The listing builds one solid part. Answer for the finished solid, in the listing's coordinates (mm). Coordinates: 2 decimals unless noted, no trailing zeros. Loops run counter-clockwise (first coordinate to the right, second up) from the corner with the lowest first, then second, coordinate; pieces in that order, holes last. Notation, with made-up numbers: (-21.5, -22.75) - (27.5, -22.75) arc R23 cw to (27.5, 5.25) - close; hole circle Ø7 at (59, -7). An arc over 180 degrees is marked (long way). Return JSON: item names as keys, results as strings. Group by question number.
1. Section B-B (y = 234.5) is taken. Write down the section's boundary in (x, z), and give its area (3 significant figures).
2. Find the intervals of material crossed by line 1 along Y through (x, z) = (152.5, 5); line 2 along X through (y, z) = (35, 3.75); line 3 along Y through (x, z) = (40, 4), in increasing order.
3. Section A-A (z = 6.5) is taken. State how many separate pieces and enclosed holes the cut face has, and give its area (3 significant figures).
4. Section C-C (x = 331) is taken. Write down the section's boundary in (y, z).
5. Each of these flat-tipped pins is pushed along its axis until it touches: P1, Ø3, axis at x = 231.5, z = 6.5, coming from the +Y side; P2, Ø2, axis at x = 375.5, z = 11, coming from the +Y side; P3, Ø6, axis at y = 74, z = 5, coming from the +X side. Where does it stop, or does it pass through?
```python
from build123d import *

# Parameters (mm, degrees)
F1_DEPTH = 12.7
F3_DEPTH = 12.701
F5_D     = 5.08


with BuildPart() as f1:
    # F0 (on Top) → F1 (new body)
    with BuildSketch(Plane.XY):
        Polygon((349.925731, -349.925731), (494.869714, 0), (349.925731, 349.925731), (0, -494.869714), align=None)
    extrude(amount=F1_DEPTH)

    # F2 (on face) → F3 (cut, through all)
    with BuildSketch(Plane.XY.offset(12.7)):
        with BuildLine():
            Line((357.632779, 298.132571), (354.903108, 299.75415))
            ThreePointArc((354.903108, 299.75415), (356.79197, 295.070926), (360.807779, 298.132571))
            ThreePointArc((360.807779, 298.132571), (360.746772, 298.751982), (360.566096, 299.347591))
            Line((360.566096, 299.347591), (357.632779, 298.132571))
        make_face()
        with BuildLine():
            ThreePointArc((360.566096, 299.347591), (357.860135, 301.29942), (354.903108, 299.75415))
            Line((354.903108, 299.75415), (357.632779, 298.132571))
            Line((357.632779, 298.132571), (360.566096, 299.347591))
        make_face()
        with BuildLine():
            Line((463.696126, 42.073001), (463.696126, 45.248001))
            ThreePointArc((463.696126, 45.248001), (461.451062, 39.827937), (466.871126, 42.073001))
            ThreePointArc((466.871126, 42.073001), (466.810119, 42.692412), (466.629443, 43.288021))
            Line((466.629443, 43.288021), (463.696126, 42.073001))
        make_face()
        with BuildLine():
            ThreePointArc((466.629443, 43.288021), (465.460061, 44.712917), (463.696126, 45.248001))
            Line((463.696126, 45.248001), (463.696126, 42.073001))
            Line((463.696126, 42.073001), (466.629443, 43.288021))
        make_face()
        with BuildLine():
            ThreePointArc((466.629443, -43.288021), (466.810119, -42.692412), (466.871126, -42.073001))
            ThreePointArc((466.871126, -42.073001), (465.94119, -39.827937), (463.696126, -38.898001))
            Line((463.696126, -38.898001), (463.696126, -42.073001))
            Line((463.696126, -42.073001), (466.629443, -43.288021))
        make_face()
        with BuildLine():
            Line((463.696126, -42.073001), (463.696126, -38.898001))
            ThreePointArc((463.696126, -38.898001), (461.05621, -43.836936), (466.629443, -43.288021))
            Line((466.629443, -43.288021), (463.696126, -42.073001))
        make_face()
        with BuildLine():
            ThreePointArc((360.566096, -299.347591), (360.746772, -298.751982), (360.807779, -298.132571))
            ThreePointArc((360.807779, -298.132571), (359.877843, -295.887507), (357.632779, -294.957571))
            Line((357.632779, -294.957571), (357.632779, -298.132571))
            Line((357.632779, -298.132571), (360.566096, -299.347591))
        make_face()
        with BuildLine():
            Line((357.632779, -298.132571), (357.632779, -294.957571))
            ThreePointArc((357.632779, -294.957571), (354.992863, -299.896506), (360.566096, -299.347591))
            Line((360.566096, -299.347591), (357.632779, -298.132571))
        make_face()
        with BuildLine():
            ThreePointArc((299.347591, -360.566096), (300.772487, -359.396714), (301.307571, -357.632779))
            ThreePointArc((301.307571, -357.632779), (300.377635, -355.387715), (298.132571, -354.457779))
            Line((298.132571, -354.457779), (298.132571, -357.632779))
            Line((298.132571, -357.632779), (299.347591, -360.566096))
        make_face()
        with BuildLine():
            Line((298.132571, -357.632779), (298.132571, -354.457779))
            ThreePointArc((298.132571, -354.457779), (295.018577, -358.252191), (299.347591, -360.566096))
            Line((299.347591, -360.566096), (298.132571, -357.632779))
        make_face()
        with BuildLine():
            ThreePointArc((43.288021, -466.629443), (44.712917, -465.460061), (45.248001, -463.696126))
            ThreePointArc((45.248001, -463.696126), (44.712917, -461.93219), (43.288021, -460.762808))
            Line((43.288021, -460.762808), (42.073001, -463.696126))
            Line((42.073001, -463.696126), (43.288021, -466.629443))
        make_face()
        with BuildLine():
            Line((42.073001, -463.696126), (43.288021, -460.762808))
            ThreePointArc((43.288021, -460.762808), (38.898001, -463.696126), (43.288021, -466.629443))
            Line((43.288021, -466.629443), (42.073001, -463.696126))
        make_face()
    extrude(amount=-F3_DEPTH, mode=Mode.SUBTRACT)

    # F5 (through all)
    with Locations(Plane.XY.offset(12.7)):
        with Locations((307.474792, 57.228103), (269.994706, -120.526589), (391.079336, 15.960708), (214.770496, -298.838586), (153.693318, -271.606386)):
            Hole(F5_D / 2)


solid = f1.part
```
The answers:
{
 "1": {"outline": "(302.11, 0) - (397.74, 0) - (397.74, 12.7) - (302.11, 12.7) - close", "area": "1,210 mm2"},
 "2": {"line 1": "y = -431.7 to -273.85, -269.36 to -126.7", "line 2": "x = 219.48 to 480.37", "line 3": "y = -478.3 to -466.1, -461.29 to -398.3"},
 "3": {"separate pieces": "1", "enclosed holes": "11", "area": "173,000 mm2"},
 "4": {"outline": "(-357.77, 0) - (304.23, 0) - (304.23, 12.7) - (-357.77, 12.7) - close"},
 "5": {"P1": "stops at y = 67.64", "P2": "stops at y = 290.6", "P3": "stops at x = 465.46"}
}
